Part model, mm, in its own coordinate system. A direction names the side the tool comes from. Coordinates: 2 decimals unless noted, no trailing zeros. Write each loop counter-clockwise with the first axis right and the second up, starting at its lowest first coordinate (ties: lowest second). Pieces come first, ordered by that corner, then holes. Notation, with made-up numbers: (70, 35.5) - (126, 35.5) arc R5 ccw to (126, 41.5) - close; hole circle Ø9 at (53.25, 7). An arc over 180 degrees is marked (long way). Use one line per item in the form item = value. Start each with the question number.
from build123d import *

# Parameters (mm, degrees)
SKETCH1_W                    = 51
SKETCH1_H                    = 51
BOSS_EXTRUDE1_DEPTH          = 30
CUT_EXTRUDE1_DEPTH           = 31
CUT_EXTRUDE2_DEPTH           = 31
SKETCH4_W                    = 30
SKETCH4_H                    = 2.067
F_9_0_9_DIAMETER_HOLE1_D     = 9
F_9_0_9_DIAMETER_HOLE1_DEPTH = 9
F_9_0_9_DIAMETER_HOLE2_D     = 9
F_9_0_9_DIAMETER_HOLE2_DEPTH = 9
CHAMFER1_SIZE                = 0.433


with BuildPart() as part:
    # Sketch1 → Boss-Extrude1 (new body)
    with BuildSketch(Plane(origin=(15, 0, 0), x_dir=(0, 0, -1), z_dir=(1, 0, 0))):
        with Locations((-25.5, 25.5)):
            Rectangle(SKETCH1_W, SKETCH1_H)
    extrude(amount=-BOSS_EXTRUDE1_DEPTH)

    # Sketch2 → Cut-Extrude1 (cut, through all)
    with BuildSketch(Plane.ZY.offset(15)):
        Polygon((9, 51), (9, 29), (29, 9), (51, 9), (51, 51), align=None)
    extrude(amount=-CUT_EXTRUDE1_DEPTH, mode=Mode.SUBTRACT)

    # Sketch3 → Cut-Extrude2 (cut, through all)
    with BuildSketch(Plane.ZY.offset(15)):
        with BuildLine():
            Line((12, 8.9), (12, 7))
            Line((12, 7), (25.757359313, 7))
            ThreePointArc((25.757359313, 7), (26.681238845, 7.617316568), (26.464466094, 8.707106781))
            Line((26.464466094, 8.707106781), (8.707106781, 26.464466094))
            ThreePointArc((8.707106781, 26.464466094), (7.617316568, 26.681238845), (7, 25.757359313))
            Line((7, 25.757359313), (7, 12))
            Line((7, 12), (8.9, 12))
            ThreePointArc((8.9, 12), (10.00735841, 14.374737774), (12.538309351, 15.052904034))
            Line((12.538309351, 15.052904034), (12.364661173, 14.068096281))
            ThreePointArc((12.364661173, 14.068096281), (11.523597358, 11.523597358), (14.068096281, 12.364661173))
            Line((14.068096281, 12.364661173), (15.052904034, 12.538309351))
            ThreePointArc((15.052904034, 12.538309351), (14.374737774, 10.00735841), (12, 8.9))
        make_face()
    extrude(amount=-CUT_EXTRUDE2_DEPTH, mode=Mode.SUBTRACT)

    # Sketch4 → Cut-Revolve1 (revolve, cut)
    with BuildSketch(Plane.XY.offset(12)):
        with Locations((0, 13.0335)):
            Rectangle(SKETCH4_W, SKETCH4_H)
    revolve(axis=Axis((-15, 12, 12), (1, 0, 0)), mode=Mode.SUBTRACT)

    # Ø9.0 (9) Diameter Hole1
    with Locations(Plane.XY.offset(9)):
        with Locations((0, 41)):
            Hole(F_9_0_9_DIAMETER_HOLE1_D / 2, depth=F_9_0_9_DIAMETER_HOLE1_DEPTH)

    # Ø9.0 (9) Diameter Hole2
    with Locations(Plane(origin=(0, 9, 0), x_dir=(1, 0, 0), z_dir=(0, 1, 0))):
        with Locations((0, -41)):
            Hole(F_9_0_9_DIAMETER_HOLE2_D / 2, depth=F_9_0_9_DIAMETER_HOLE2_DEPTH)

    # Chamfer1
    chamfer1_edges = [part.edges().sort_by_distance(p)[0] for p in [
        (15, 14.059848355, 12.31475481),
        (15, 10.538410283, 10.538410283),
    ]]
    chamfer(chamfer1_edges, length=CHAMFER1_SIZE)


solid = part.part
Q1. Slice it at D-D (z = 5). List the corners of the cut face in (x, y), plus the area to 3 significant figures.
Q2. Mould opens along X. For faces 4 (the flat face through (0, 0, 26)), 5 (the cylindrical face through (0.98, 4.44, 45.39)), 6 (the flat face through (-15, 18, 18)) say: released by +X, released by -X, zero draft, split by the parting line, or undercut.
Q3. Which spindle directions (+Z, -Z, +X, -X, +Y, -Y) get a long thin tool onto all of the face, cutting with end or side? Do faces 1 (the flat face through (0, 51, 5)), 2 (the flat face through (-4, 9, 37)), 3 (the cylindrical face through (-0.21, 14.35, 9.98)). Say none if no direction does.
Q4. Slice it at A-A (z = 41). List the corners of the cut face in (x, y).
Q5. Drill centre lines: probe 1 along Z at (x, y) = (0, 5); probe 2 along Z at (x, y) = (-3, 8.5). Where is each one in solid material? Low to high.
Q6. Pin check, flat tips, straight feed: P1, Ø7, axis at x = -1.5, z = 19, coming from the +Y side; P2, Ø10, axis at x = -4, z = 38.5, coming from the +Y side; P3, Ø11, axis at x = -4.5, y = 21.5, coming from the +Z side; P4, Ø3.5, axis at y = 12, z = 12, coming from the -X side. Stop position of each tip, or through.
Q7. Slice it at B-B (x = -11.5). List the corners of the cut face in (y, z).
Solution:
q1.outline = (-15, 0) - (15, 0) - (15, 51) - (-15, 51) - close; hole circle Ø9 at (0, 41)
q1.area = 1,470 mm2
q2.face_4 = zero draft
q2.face_5 = undercut
q2.face_6 = released by -X
q3.face_1 = +Z, -Z, +X, -X, +Y
q3.face_2 = +Z, +X, -X, +Y
q3.face_3 = +X, -X
q4.outline = (-15, 0) - (-4.5, 0) - (-4.5, 9) - (-15, 9) - close; (4.5, 0) - (15, 0) - (15, 9) - (4.5, 9) - close
q5.probe_1 = 0 to 36.5, 45.5 to 51
q5.probe_2 = 0 to 12, 26.62 to 37.65, 44.35 to 51
q6.P1 = 22.5
q6.P2 = 9
q6.P3 = 22
q6.P4 = through
q7.outline = (0, 0) - (51, 0) - (51, 9) - (29, 9) - (9, 29) - (9, 51) - (0, 51) - close; hole (7, 12) - (8.9, 12) arc R3.1 cw to (12.54, 15.05) - (12.36, 14.07) arc R1.5 ccw to (12.27, 14.05) arc R2.07 ccw (long way) to (14.05, 12.27) arc R1.5 ccw to (14.07, 12.36) - (15.05, 12.54) arc R3.1 cw to (12, 8.9) - (12, 7) - (25.76, 7) arc R1 ccw to (26.46, 8.71) - (8.71, 26.46) arc R1 ccw to (7, 25.76) - close
